Read the model definition and answer for the solid it produces. Units are mm, in the model's axes. Face numbers are marked on the shaded views. A direction names the side the tool comes from. Round coordinates to 2 decimals unless told otherwise and drop trailing zeros. Write each loop counter-clockwise with the first axis right and the second up, starting at its lowest first coordinate (ties: lowest second). Pieces come first, ordered by that corner, then holes. Notation, with made-up numbers: (-8, 20) -> (8, 20) arc R21 ccw to (8, 33) -> close; hole circle Ø2 at (19, -39). An arc over 180 degrees is marked (long way). Return JSON: item names as keys, results as strings.
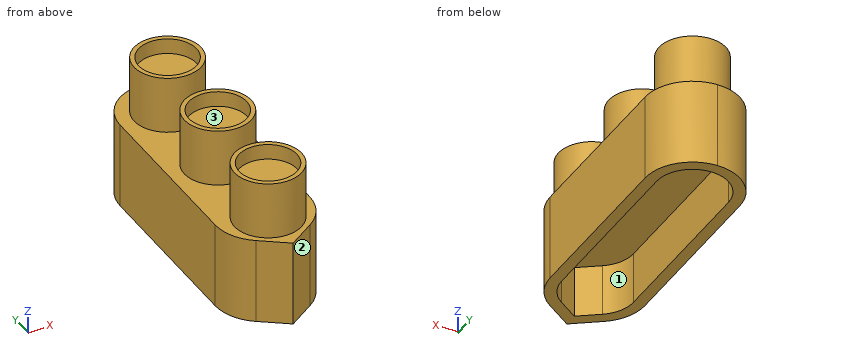
from build123d import *
from OCP.BRepFilletAPI import BRepFilletAPI_MakeChamfer

# Parameters (mm, degrees)
SKETCH1_W                       = 16.5
SKETCH1_H                       = 49.5
BOSS_EXTRUDE1_DEPTH             = 25
SKETCH2_R                       = 5.85
SKETCH2_R_2                     = 5.05
CUT_EXTRUDE1_DEPTH              = 10
FILLET5_R                       = 8.25
CHAMFER1_SIZE                   = 5.77671219
CHAMFER1_SIZE_2                 = 8.25
FILLET6_R                       = 8.25
SKETCH4_R                       = 5.1
BOSS_EXTRUDE2_DEPTH             = 7.3
SCHNITT_LINEAR_AUSTRAGEN1_DEPTH = 9


with BuildPart() as part:
    # Sketch1 → Boss-Extrude1 (new body)
    with BuildSketch(Plane.XY):
        with Locations((-90.75, 140.25)):
            Rectangle(SKETCH1_W, SKETCH1_H)
    extrude(amount=BOSS_EXTRUDE1_DEPTH)

    # Sketch2 → Cut-Extrude1 (cut)
    # profile 1 of 8: a face of its own
    with BuildSketch(Plane.XY.offset(25)):
        with BuildLine():
            ThreePointArc((-96.6, 140.25), (-90.75, 146.1), (-84.9, 140.25))
            Line((-84.9, 140.25), (-82.5, 140.25))
            Line((-82.5, 140.25), (-82.5, 165))
            Line((-82.5, 165), (-99, 165))
            Line((-99, 165), (-99, 140.25))
            Line((-99, 140.25), (-96.6, 140.25))
        make_face()
        with Locations((-90.75, 156.75)):
            Circle(SKETCH2_R, mode=Mode.SUBTRACT)
    # profile 2 of 8: a face of its own
    with BuildSketch(Plane.XY.offset(25)):
        with BuildLine():
            Line((-82.5, 140.25), (-84.9, 140.25))
            ThreePointArc((-84.9, 140.25), (-90.75, 134.4), (-96.6, 140.25))
            Line((-96.6, 140.25), (-99, 140.25))
            Line((-99, 140.25), (-99, 115.5))
            Line((-99, 115.5), (-82.5, 115.5))
            Line((-82.5, 115.5), (-82.5, 140.25))
        make_face()
        with Locations((-90.75, 123.75)):
            Circle(SKETCH2_R, mode=Mode.SUBTRACT)
    # profile 3 of 8: a face of its own
    with BuildSketch(Plane.XY.offset(25)):
        with BuildLine():
            ThreePointArc((-95.8, 140.25), (-90.75, 135.2), (-85.7, 140.25))
            Line((-85.7, 140.25), (-95.8, 140.25))
        make_face()
    # profile 4 of 8: a face of its own
    with BuildSketch(Plane.XY.offset(25)):
        with BuildLine():
            Line((-95.8, 140.25), (-85.7, 140.25))
            ThreePointArc((-85.7, 140.25), (-90.75, 145.3), (-95.8, 140.25))
        make_face()
    # profile 5 of 8: a face of its own
    with BuildSketch(Plane.XY.offset(25)):
        with BuildLine():
            ThreePointArc((-95.8, 140.25), (-90.75, 135.2), (-85.7, 140.25))
            Line((-85.7, 140.25), (-95.8, 140.25))
        make_face()
    # profile 6 of 8: a face of its own
    with BuildSketch(Plane.XY.offset(25)):
        with BuildLine():
            Line((-95.8, 140.25), (-85.7, 140.25))
            ThreePointArc((-85.7, 140.25), (-90.75, 145.3), (-95.8, 140.25))
        make_face()
    # profile 7 of 8: a face of its own
    with BuildSketch(Plane.XY.offset(25)):
        with Locations((-90.75, 123.75)):
            Circle(SKETCH2_R_2)
    # profile 8 of 8: a face of its own
    with BuildSketch(Plane.XY.offset(25)):
        with Locations((-90.75, 156.75)):
            Circle(SKETCH2_R_2)
    extrude(amount=-CUT_EXTRUDE1_DEPTH, mode=Mode.SUBTRACT)

    # Fillet5
    fillet5_edges = [part.edges().sort_by_distance(p)[0] for p in [
        (-82.5, 165, 7.5),
        (-99, 165, 7.5),
    ]]
    fillet(fillet5_edges, radius=FILLET5_R - 0.0001)  # a hair under: the kernel refuses the full size

    # Chamfer1
    chamfer1_edges_1 = [part.edges().sort_by_distance(p)[0] for p in [
        (-99, 115.5, 7.5),
    ]]
    chamfer1_side_1 = [part.faces().sort_by_distance(p)[0] for p in [
        (-99, 115.615534244, 7.5),
    ]]
    chamfer1_edges_2 = [part.edges().sort_by_distance(p)[0] for p in [
        (-82.5, 115.5, 7.5),
    ]]
    chamfer1_side_2 = [part.faces().sort_by_distance(p)[0] for p in [
        (-82.5, 115.615534244, 7.5),
    ]]
    chamfer1 = BRepFilletAPI_MakeChamfer(part.part.solid().wrapped)
    for e in chamfer1_edges_1:
        chamfer1.Add(CHAMFER1_SIZE - 0.0001, CHAMFER1_SIZE_2 - 0.0001, e.wrapped, chamfer1_side_1[0].wrapped)
    for e in chamfer1_edges_2:
        chamfer1.Add(CHAMFER1_SIZE - 0.0001, CHAMFER1_SIZE_2 - 0.0001, e.wrapped, chamfer1_side_2[0].wrapped)
    add(Compound.cast(chamfer1.Shape()), mode=Mode.REPLACE)  # a hair under: the kernel refuses the full size

    # Fillet6
    fillet6_edges = [part.edges().sort_by_distance(p)[0] for p in [
        (-99, 121.27661219, 7.5),
        (-82.5, 121.27661219, 7.5),
    ]]
    fillet(fillet6_edges, radius=FILLET6_R)

    # Sketch4 → Boss-Extrude2 (add)
    with BuildSketch(Plane.XY.offset(15)):
        with Locations((-90.75, 156.75)):
            Circle(SKETCH4_R)
        with Locations((-90.75, 140.25)):
            Circle(SKETCH4_R)
        with Locations((-90.75, 123.75)):
            Circle(SKETCH4_R)
    extrude(amount=BOSS_EXTRUDE2_DEPTH)

    # Skizze2 → Schnitt-Linear austragen1 (cut)
    with BuildSketch(Plane(origin=(0, 0, 0), x_dir=(-1, 0, 0), z_dir=(0, 0, -1))):
        with BuildLine():
            Line((84.5, 156.75), (84.5, 125.571390357))
            ThreePointArc((84.5, 125.571390357), (85.206182293, 122.685461525), (87.165147273, 120.45169008))
            Line((87.165147273, 120.45169008), (90.75, 117.941549178))
            Line((90.75, 117.941549178), (94.334852727, 120.45169008))
            ThreePointArc((94.334852727, 120.45169008), (96.293817707, 122.685461525), (97, 125.571390357))
            Line((97, 125.571390357), (97, 156.75))
            ThreePointArc((97, 156.75), (95.169417382, 161.169417382), (90.75, 163))
            ThreePointArc((90.75, 163), (86.330582618, 161.169417382), (84.5, 156.75))
        make_face()
    extrude(amount=-SCHNITT_LINEAR_AUSTRAGEN1_DEPTH, mode=Mode.SUBTRACT)


solid = part.part
Item 1: Section C-C (y = 123.75) is taken. Give the vertices of the cut face in (x, z), then the cut area to 3 significant figures.
Worked answers:
{"outline": "(-98.8, 0) -> (-96.73, 0) -> (-96.73, 9) -> (-84.77, 9) -> (-84.77, 0) -> (-82.7, 0) -> (-82.7, 15) -> (-84.9, 15) -> (-84.9, 25) -> (-85.7, 25) -> (-85.7, 22.3) -> (-95.8, 22.3) -> (-95.8, 25) -> (-96.6, 25) -> (-96.6, 15) -> (-98.8, 15) -> close", "area": "224 mm2"}
Item 2: A tool of negligible diameter and unlimited length cuts with its end or side. For the marked faces 1, 2 and 3, from which of +Z, -Z, +X, -X, +Y, -Y can it reach the whole face along a straight path? Write none if from no direction.
Worked answers:
{"face 1": "-Z", "face 2": "+Z, -Z, +X, -Y", "face 3": "+Z"}
Item 3: Section A-A (z = 23) is taken. Give the vertices of the cut face in (x, y).
Worked answers:
{"outline": "circle Ø11.7 at (-90.75, 123.75); circle Ø11.7 at (-90.75, 140.25); circle Ø11.7 at (-90.75, 156.75); hole circle Ø10.1 at (-90.75, 123.75); hole circle Ø10.1 at (-90.75, 140.25); hole circle Ø10.1 at (-90.75, 156.75)"}
Item 4: Section D-D (z = 15.75) is taken. Give the vertices of the cut face in (x, y), then the cut area to 3 significant figures.
Worked answers:
{"outline": "circle Ø11.7 at (-90.75, 123.75); circle Ø11.7 at (-90.75, 140.25); circle Ø11.7 at (-90.75, 156.75)", "area": "323 mm2"}
Item 5: Flat-ended cylindrical pins translate along their axes: pin 1 (3 mm diameter, centred on x = -93, y = 125.5, fed in from +Z); pin 2 (3 mm diameter, centred on x = -91, z = 22.5, fed in from -Y); pin 3 (3 mm diameter, centred on x = -84.5, z = 7, fed in from +Y). Find the tip coordinate at first contact, or state that the pin passes through.
Worked answers:
{"pin 1": "stops at z = 22.3", "pin 2": "stops at y = 117.9", "pin 3": "stops at y = 163.5"}
Item 6: Straight lines are drawn through the part: L1, parallel to Y at x = -90.75, z = 23.15; L2, parallel to Y at x = -93.75, z = 20; L3, parallel to Y at x = -88, z = 17. For each, find the intervals that lie inside material, in ascending order. Write a range as [from, to].
Worked answers:
{"L1": "y = [117.9, 118.7], [128.8, 129.6], [134.4, 135.2], [145.3, 146.1], [150.9, 151.7], [161.8, 162.6]", "L2": "y = [118.73, 128.77], [135.23, 145.27], [151.73, 161.77]", "L3": "y = [118.59, 128.91], [135.09, 145.41], [151.59, 161.91]"}
